Geometry: final body of the model. Coordinates: model frame, mm. A direction names the side the tool comes from. Round coordinates to 2 decimals unless told otherwise and drop trailing zeros. Loops run counter-clockwise (first coordinate to the right, second up) from the corner with the lowest first, then second, coordinate; pieces in that order, holes last. Notation, with made-up numbers: (-39, 21.5) - (-6, 21.5) arc R18 ccw to (-6, 37.5) - close; hole circle Ø10 at (-3.75, 12.5). An arc over 180 degrees is marked (long way). Return JSON: item names as keys, results as strings. Group by question number.
1. Section C-C on y = 18.5. Return loops of the section in (x, z).
2. Set-up query: faces 1 (the face through (6.6, 6, 23)), 2 (the face through (8, 20.5, 5)), 3 (the face through (6.02, 5.19, 42.46)). Return all of +Z, -Z, +X, -X, +Y, -Y with unobstructed straight access to the full face (end or side cutting, diameter ignored); none if empty.
3. Section A-A on z = 22.5. Return loops of the section in (x, y), and give its area (4 significant figures).
4. Section B-B on y = 28.8. Return loops of the section in (x, z).
5. Material intervals for probe 1 along Y at (x, z) = (1.7, 5); probe 2 along Y at (x, z) = (2.7, 40); probe 3 along Z at (x, y) = (3.75, 2.1), sorted ascending.
6. Draft query along Y for faces 4 (the face through (5, 4.5, 24)), 5 (the face through (6, 0.9, 5)), 6 (the face through (0.9, 6, 22)). Return one class per face: +Y half, -Y half, draft (parallel to the pull), parting line (faces both ways), or undercut.
7. Section D-D on z = 14. Return loops of the section in (x, y), and give its area (4 significant figures).
8. First-contact query: pin 1 Ø3 at (x, y) = (9.5, 17) entering from +Z; pin 2 Ø6 at (x, z) = (8.5, 24) entering from +Y; pin 3 Ø0.9 at (y, z) = (5.5, 23) entering from -X; pin 4 Ø2.5 at (y, z) = (15, 5.5) entering from -X. Flat tips, straight axial feed; report the tip coordinate or a pass-through.
from build123d import *

# Parameters (mm, degrees)
SALIENTE_EXTRUIR1_DEPTH = 4
SALIENTE_EXTRUIR2_DEPTH = 3
CROQUIS3_W              = 7.5
CROQUIS3_H              = 7.5
SALIENTE_EXTRUIR3_DEPTH = 38
CORTAR_EXTRUIR1_REACH   = 7
CROQUIS4_R              = 1.6
CORTAR_EXTRUIR2_DEPTH   = 3
CORTAR_EXTRUIR3_REACH   = 19.4
CROQUIS6_R              = 1.6
CORTAR_EXTRUIR4_DEPTH   = 3
CORTAR_EXTRUIR5_REACH   = 51.7
CROQUIS8_R              = 1.6
CORTAR_EXTRUIR6_DEPTH   = 3
CORTAR_EXTRUIR7_REACH   = 14.4
CROQUIS10_W             = 3
CROQUIS10_H             = 3.5


with BuildPart() as part:
    # Croquis1 → Saliente-Extruir1 (new body)
    with BuildSketch(Plane.XY):
        Polygon((0, 26.5), (0, 0), (7.5, 0), (7.5, 12.6), (17.4, 22.5), (17.4, 49.7), (6.2, 49.7), (6.2, 44.7), (9.2, 44.7), (9.2, 46.7), (12.4, 46.7), (12.4, 26.5), align=None)
    extrude(amount=SALIENTE_EXTRUIR1_DEPTH)

    # Croquis2 → Saliente-Extruir2 (add)
    with BuildSketch(Plane.XY.offset(4)):
        Polygon((0, 0), (0, 10.2), (5, 10.2), (5, 20.5), (0, 20.5), (0, 26.5), (12.4, 26.5), (12.4, 46.7), (9.2, 46.7), (9.2, 44.7), (6.2, 44.7), (6.2, 49.7), (17.4, 49.7), (17.4, 22.5), (7.5, 12.6), (7.5, 0), align=None)
    extrude(amount=SALIENTE_EXTRUIR2_DEPTH)

    # Croquis3 → Saliente-Extruir3 (add)
    with BuildSketch(Plane.XY.offset(7)):
        with Locations((3.75, 3.75)):
            Rectangle(CROQUIS3_W, CROQUIS3_H)
    extrude(amount=SALIENTE_EXTRUIR3_DEPTH)

    # Croquis4 → Cortar-Extruir1 (cut, up to next)
    with BuildSketch(Plane.ZY.offset(-12.4), mode=Mode.PRIVATE) as cortar_extruir1_sk1:
        with Locations((3.5, 28.8)):
            Circle(CROQUIS4_R)
    cortar_extruir1_tool1 = extrude(cortar_extruir1_sk1.sketch, amount=-CORTAR_EXTRUIR1_REACH, mode=Mode.PRIVATE) & part.part
    add(cortar_extruir1_tool1.solids().sort_by_distance((12.4, 28.8, 3.5))[0], mode=Mode.SUBTRACT)

    # Croquis5 → Cortar-Extruir2 (cut)
    with BuildSketch(Plane(origin=(17.4, 0, 0), x_dir=(0, 0, -1), z_dir=(1, 0, 0))):
        Polygon((-0.65, 30.445448267), (-3.5, 32.090896534), (-6.35, 30.445448267), (-6.35, 27.154551733), (-3.5, 25.509103466), (-0.65, 27.154551733), align=None)
    extrude(amount=-CORTAR_EXTRUIR2_DEPTH, mode=Mode.SUBTRACT)

    # Croquis6 → Cortar-Extruir3 (cut, up to next)
    with BuildSketch(Plane.ZY, mode=Mode.PRIVATE) as cortar_extruir3_sk1:
        with Locations((5, 3.75)):
            Circle(CROQUIS6_R)
    cortar_extruir3_tool1 = extrude(cortar_extruir3_sk1.sketch, amount=-CORTAR_EXTRUIR3_REACH, mode=Mode.PRIVATE) & part.part
    add(cortar_extruir3_tool1.solids().sort_by_distance((0, 3.75, 5))[0], mode=Mode.SUBTRACT)
    # Croquis6 → Cortar-Extruir3 (cut, up to next)
    with BuildSketch(Plane.ZY, mode=Mode.PRIVATE) as cortar_extruir3_sk2:
        with Locations((40, 3.75)):
            Circle(CROQUIS6_R)
    cortar_extruir3_tool2 = extrude(cortar_extruir3_sk2.sketch, amount=-CORTAR_EXTRUIR3_REACH, mode=Mode.PRIVATE) & part.part
    add(cortar_extruir3_tool2.solids().sort_by_distance((0, 3.75, 40))[0], mode=Mode.SUBTRACT)

    # Croquis7 → Cortar-Extruir4 (cut)
    with BuildSketch(Plane(origin=(7.5, 0, 0), x_dir=(0, 0, -1), z_dir=(1, 0, 0))):
        Polygon((-3.354551733, 6.6), (-6.645448267, 6.6), (-8.290896534, 3.75), (-6.645448267, 0.9), (-3.354551733, 0.9), (-1.709103466, 3.75), align=None)
        Polygon((-38.354551733, 6.6), (-41.645448267, 6.6), (-43.290896534, 3.75), (-41.645448267, 0.9), (-38.354551733, 0.9), (-36.709103466, 3.75), align=None)
    extrude(amount=-CORTAR_EXTRUIR4_DEPTH, mode=Mode.SUBTRACT)

    # Croquis8 → Cortar-Extruir5 (cut, up to next)
    with BuildSketch(Plane.XZ, mode=Mode.PRIVATE) as cortar_extruir5_sk1:
        with Locations((3.75, 22.5)):
            Circle(CROQUIS8_R)
    cortar_extruir5_tool1 = extrude(cortar_extruir5_sk1.sketch, amount=-CORTAR_EXTRUIR5_REACH, mode=Mode.PRIVATE) & part.part
    add(cortar_extruir5_tool1.solids().sort_by_distance((3.75, 0, 22.5))[0], mode=Mode.SUBTRACT)

    # Croquis9 → Cortar-Extruir6 (cut)
    with BuildSketch(Plane(origin=(0, 7.5, 0), x_dir=(1, 0, 0), z_dir=(0, 1, 0))):
        Polygon((0.9, -20.854551733), (0.9, -24.145448267), (3.75, -25.790896534), (6.6, -24.145448267), (6.6, -20.854551733), (3.75, -19.209103466), align=None)
    extrude(amount=-CORTAR_EXTRUIR6_DEPTH, mode=Mode.SUBTRACT)

    # Croquis10 → Cortar-Extruir7 (cut, up to next)
    with BuildSketch(Plane.ZY.offset(-5), mode=Mode.PRIVATE) as cortar_extruir7_sk1:
        with Locations((5.5, 11.95)):
            Rectangle(CROQUIS10_W, CROQUIS10_H)
    cortar_extruir7_tool1 = extrude(cortar_extruir7_sk1.sketch, amount=-CORTAR_EXTRUIR7_REACH, mode=Mode.PRIVATE) & part.part
    add(cortar_extruir7_tool1.solids().sort_by_distance((5, 11.95, 5.5))[0], mode=Mode.SUBTRACT)
    # Croquis10 → Cortar-Extruir7 (cut, up to next)
    with BuildSketch(Plane.ZY.offset(-5), mode=Mode.PRIVATE) as cortar_extruir7_sk2:
        with Locations((5.5, 18.75)):
            Rectangle(CROQUIS10_W, CROQUIS10_H)
    cortar_extruir7_tool2 = extrude(cortar_extruir7_sk2.sketch, amount=-CORTAR_EXTRUIR7_REACH, mode=Mode.PRIVATE) & part.part
    add(cortar_extruir7_tool2.solids().sort_by_distance((5, 18.75, 5.5))[0], mode=Mode.SUBTRACT)


solid = part.part
Taken from the geometry:
{
 "1": {"outline": "(0, 0) - (13.4, 0) - (13.4, 4) - (0, 4) - close"},
 "2": {"face 1": "+Y", "face 2": "+Z, +X, -X", "face 3": "+X"},
 "3": {"outline": "(0, 0) - (2.15, 0) - (2.15, 4.5) - (0.9, 4.5) - (0.9, 7.5) - (0, 7.5) - close; (5.35, 0) - (7.5, 0) - (7.5, 7.5) - (6.6, 7.5) - (6.6, 4.5) - (5.35, 4.5) - close", "area": "24.75 mm2"},
 "4": {"outline": "(12.4, 0) - (17.4, 0) - (17.4, 0.65) - (14.4, 0.65) - (14.4, 1.9) - (12.4, 1.9) - close; (12.4, 5.1) - (14.4, 5.1) - (14.4, 6.35) - (17.4, 6.35) - (17.4, 7) - (12.4, 7) - close"},
 "5": {"probe 1": "0 to 2.15, 5.35 to 10.2, 20.5 to 26.5", "probe 2": "0 to 2.15, 5.35 to 7.5", "probe 3": "0 to 20.9, 24.1 to 45"},
 "6": {"face 4": "+Y half", "face 5": "undercut", "face 6": "draft"},
 "7": {"outline": "(0, 0) - (7.5, 0) - (7.5, 7.5) - (0, 7.5) - close", "area": "56.25 mm2"},
 "8": {"pin 1": "z = 7", "pin 2": "y = 7.5", "pin 3": "x = 0", "pin 4": "x = 5"}
}
